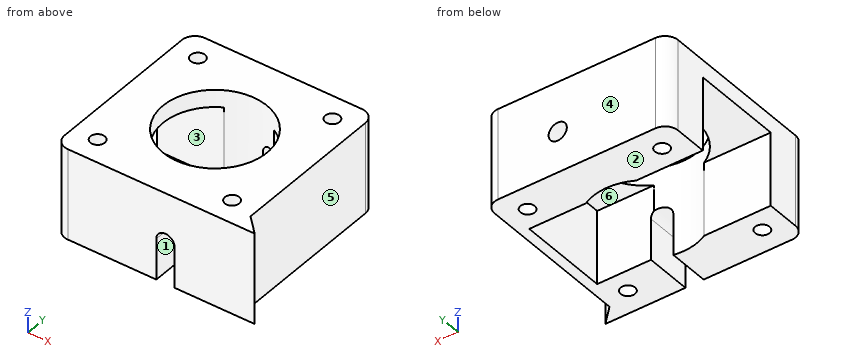
from build123d import *

# Parameters (mm, degrees)
IZIM1_R                     = 1.65
Y_KSEKLIK_EKSTR_ZYON1_DEPTH = 21
RADYUS1_R                   = 3
IZIM4_W                     = 17
IZIM4_H                     = 21
KES_EKSTR_ZYON3_DEPTH       = 40
IZIM5_R                     = 2.1
KES_EKSTR_ZYON4_DEPTH       = 55
IZIM2_R                     = 12
KES_EKSTR_ZYON1_DEPTH       = 10
KES_EKSTR_ZYON1_DEPTH_BACK  = 23
KES_EKSTR_ZYON5_DEPTH       = 15


with BuildPart() as part:
    # Çizim1 → Yükseklik-Ekstrüzyon1 (new body)
    with BuildSketch(Plane.XY):
        Polygon((-6.954216705, -22.021401373), (-4.12578958, -22.021401373), (7.545783295, -22.021401373), (10.37421042, -22.021401373), (18.259996857, -22.021401373), (22.019996857, -22.021401373), (18.259996857, -18.261401373), (18.259996857, 20.278598627), (-24.040003143, 20.278598627), (-24.040003143, -22.021401373), align=None)
        with Locations((-18.390003143, 14.628598627)):
            Circle(IZIM1_R, mode=Mode.SUBTRACT)
        with Locations((12.609996857, 14.628598627)):
            Circle(IZIM1_R, mode=Mode.SUBTRACT)
        with Locations((-18.390003143, -16.371401373)):
            Circle(IZIM1_R, mode=Mode.SUBTRACT)
        with Locations((12.609996857, -16.371401373)):
            Circle(IZIM1_R, mode=Mode.SUBTRACT)
    extrude(amount=Y_KSEKLIK_EKSTR_ZYON1_DEPTH)

    # Radyus1
    radyus1_edges = [part.edges().sort_by_distance(p)[0] for p in [
        (-24.040003143, 20.278598627, 10.5),
        (18.259996857, 20.278598627, 10.5),
        (-24.040003143, -22.021401373, 10.5),
    ]]
    fillet(radyus1_edges, radius=RADYUS1_R)

    # Çizim4 → Kes-Ekstrüzyon3 (cut)
    with BuildSketch(Plane.ZY.offset(24.040003143)):
        with Locations((8.5, -0.871401373)):
            Rectangle(IZIM4_W, IZIM4_H)
    extrude(amount=-KES_EKSTR_ZYON3_DEPTH, mode=Mode.SUBTRACT)

    # Çizim5 → Kes-Ekstrüzyon4 (cut)
    with BuildSketch(Plane(origin=(0, 20.278598627, 0), x_dir=(1, 0, 0), z_dir=(0, 1, 0))):
        with Locations((1.459996857, -9.5)):
            Circle(IZIM5_R)
    extrude(amount=-KES_EKSTR_ZYON4_DEPTH, mode=Mode.SUBTRACT)

    # Çizim2 → Kes-Ekstrüzyon1 (cut, two sides)
    with BuildSketch(Plane(origin=(0, 0, 0), x_dir=(-1, 0, 0), z_dir=(0, 0, -1))) as kes_ekstr_zyon1_sk:
        with Locations((2.890003143, -0.871401373)):
            Circle(IZIM2_R)
    extrude(amount=KES_EKSTR_ZYON1_DEPTH, mode=Mode.SUBTRACT)
    extrude(kes_ekstr_zyon1_sk.sketch, amount=-KES_EKSTR_ZYON1_DEPTH_BACK, mode=Mode.SUBTRACT)

    # Çizim6 → Kes-Ekstrüzyon5 (cut)
    with BuildSketch(Plane.XZ.offset(22.021401373)):
        with BuildLine():
            Line((-0.640003143, 9.5), (-0.640003143, 0))
            Line((-0.640003143, 0), (3.559996857, 0))
            Line((3.559996857, 0), (3.559996857, 9.5))
            ThreePointArc((3.559996857, 9.5), (1.459996857, 11.6), (-0.640003143, 9.5))
        make_face()
    extrude(amount=-KES_EKSTR_ZYON5_DEPTH, mode=Mode.SUBTRACT)


solid = part.part
The listing builds one solid part. Answer for the finished solid, in the listing's coordinates (mm). Face numbers are marked on the shaded views. A direction names the side the tool comes from. Round coordinates to 2 decimals unless told otherwise and drop trailing zeros. Order: outer loops, then holes, each group sorted by start corner. A loop starts at its lowest first (then second) coordinate and runs counter-clockwise, first axis right, second up. Notation, with made-up numbers: M -5.5,65 L 10.5,65 A18 cw 10.5,84 Z; hole C 25.5,79.5 d4. An arc over 180 degrees is marked long. Answer in a Markdown table with one row per item. Add a question column.
1) The part is cut by section A-A on z = 6.25. Determine the outline of the cut face in (x, y), plus the area to 3 significant figures.
2) Consider line 1 along Y through (x, z) = (-18.5, 15.75); line 2 along Y through (x, z) = (13.5, 18); line 3 along X through (y, z) = (14, 11.75). Determine where each line is inside the solid, lowest interval first. Write a range as from..to.
3) Determine the mould class of the marked faces 4, 5 and 6 for opening direction Y: pulls with the +Y half, pulls with the -Y half, needs draft (parallel to the pull), parting line crosses it, or undercut.
4) The part is cut by section D-D on x = -4. Determine the outline of the cut face in (y, z), plus the area to 3 significant figures.
5) The part is cut by section C-C on x = -16. Determine the outline of the cut face in (y, z), plus the area to 3 significant figures.
6) Which of the six approach directions +Z, -Z, +X, -X, +Y, -Y give full straight-line access (tool end or side, diameter ignored) to the marked faces 1, 2 and 3?
7) Flat-ended cylindrical pins translate along their axes: pin 1 Ø19 at (x, y) = (-2.89, -0.87) entering from -Z; pin 2 Ø10.5 at (y, z) = (-7, 15) entering from +X; pin 3 Ø5 at (x, y) = (-19, -5.5) entering from -Z; pin 4 Ø10 at (y, z) = (-4, 6) entering from -X. Find the tip coordinate at first contact, or state that the pin passes through.
8) The part is cut by section B-B on y = 9. Determine the outline of the cut face in (x, z), plus the area to 3 significant figures.
Findings below:
| question | item | result |
|---|---|---|
| 1 | outline | M -24.04,-19.02 A3 ccw -21.04,-22.02 L -0.64,-22.02 L -0.64,-12.66 A12 cw -8.7,-11.37 L -24.04,-11.37 Z; M -24.04,9.63 L -8.7,9.63 A12 cw 2.92,9.63 L 15.96,9.63 L 15.96,-11.37 L 3.56,-11.37 L 3.56,-22.02 L 22.02,-22.02 L 18.26,-18.26 L 18.26,17.28 A3 ccw 15.26,20.28 L -21.04,20.28 A3 ccw -24.04,17.28 Z; hole C -18.39,-16.37 d3.3; hole C -18.39,14.63 d3.3; hole C 12.61,-16.37 d3.3; hole C 12.61,14.63 d3.3 |
| 1 | area | 851 mm² |
| 2 | line 1 | y = -22.02..-18.02, -14.73..-11.37, 9.63..12.98, 16.27..20.28 |
| 2 | line 2 | y = -22.02..-17.76, -14.98..13.24, 16.02..20.28 |
| 2 | line 3 | x = -24.04..-19.92, -16.86..11.08, 14.14..18.26 |
| 3 | face 4 | pulls with the +Y half |
| 3 | face 5 | needs draft |
| 3 | face 6 | undercut |
| 4 | outline | M -22.02,0 L -12.82,0 L -12.82,21 L -22.02,21 Z; M 11.08,0 L 20.28,0 L 20.28,21 L 11.08,21 Z |
| 4 | area | 386 mm² |
| 5 | outline | M -22.02,0 L -11.37,0 L -11.37,17 L 9.63,17 L 9.63,0 L 20.28,0 L 20.28,21 L -22.02,21 Z |
| 5 | area | 531 mm² |
| 6 | face 1 | -Z, -Y |
| 6 | face 2 | -Z, +X, -X, +Y, -Y |
| 6 | face 3 | -Z, -X |
| 7 | pin 1 | passes through |
| 7 | pin 2 | stops at x = 18.26 |
| 7 | pin 3 | stops at z = 17 |
| 7 | pin 4 | stops at x = 15.96 |
| 8 | outline | M -24.04,17 L -9.71,17 L -9.71,21 L -24.04,21 Z; M 3.93,17 L 15.96,17 L 15.96,0 L 18.26,0 L 18.26,21 L 3.93,21 Z |
| 8 | area | 154 mm² |
